from build123d import *

# Parameters (mm, degrees)
SKETCH2_W           = 236.22
SKETCH2_H           = 203.2
BOSS_EXTRUDE1_DEPTH = 3.175
SKETCH3_W           = 236.22
SKETCH3_H           = 3.175
BOSS_EXTRUDE2_DEPTH = 127
FILLET1_R           = 3.175
FILLET2_R           = 6.35


with BuildPart() as part:
    # Sketch2 → Boss-Extrude1 (new body)
    with BuildSketch(Plane.XY):
        Rectangle(SKETCH2_W, SKETCH2_H)
    extrude(amount=BOSS_EXTRUDE1_DEPTH)

    # Sketch3 → Boss-Extrude2 (add)
    with BuildSketch(Plane.XY.offset(3.175)):
        with Locations((0, -100.0125)):
            Rectangle(SKETCH3_W, SKETCH3_H)
    extrude(amount=BOSS_EXTRUDE2_DEPTH)

    # Fillet1
    fillet1_edges = [part.edges().sort_by_distance(p)[0] for p in [
        (0, -98.425, 3.175),
        (0, -101.6, 0),
    ]]
    fillet(fillet1_edges, radius=FILLET1_R)

    # Fillet2
    fillet2_edges = [part.edges().sort_by_distance(p)[0] for p in [
        (-118.11, -100.0125, 130.175),
        (118.11, -100.0125, 130.175),
        (-118.11, 101.6, 1.5875),
        (118.11, 101.6, 1.5875),
    ]]
    fillet(fillet2_edges, radius=FILLET2_R)


solid = part.part
Geometry: final body of the model. Coordinates: model frame, mm. A direction names the side the tool comes from. Give positions to 0.01 mm unless a question says otherwise; leave off trailing zeros. Write each loop counter-clockwise with the first axis right and the second up, starting at its lowest first coordinate (ties: lowest second). Pieces come first, ordered by that corner, then holes.
(1) Cut plane C-C, the plane y = 26.5. Return loops of the section in (x, z) (3 decimals).
(2) Cut plane B-B, the plane z = 23. Return loops of the section in (x, y) (3 decimals).
(3) Access query for faces 1 (the flat face through (-2, 5, 3.175)), 2 (the flat face through (118.11, -4, 2)). Directions: +Z, -Z, +X, -X, +Y, -Y. A direction counts if a zero-diameter tool reaches every point of the face in a straight line with its end or side. Return the directions, or none.
(4) First-contact query: P1, Ø2, axis at x = -10.5, z = 98, coming from the +Y side (3 decimals); P2, Ø2, axis at x = -25.5, y = 37.5, coming from the +Z side (3 decimals). Flat tips, straight axial feed; report the tip coordinate or a pass-through.
(5) Ray query, line 1 (Z direction, x = 91, y = -19) (3 decimals); line 2 (Y direction, x = 50.5, z = 90.5) (3 decimals). Return the intervals inside material, ascending.
(6) Cut plane A-A, the plane x = -34.5. Return loops of the section in (y, z) (3 decimals), then the cut area to 3 significant figures.
Values follow:
1. outline: (-118.11, 0) - (118.11, 0) - (118.11, 3.175) - (-118.11, 3.175) - close
2. outline: (-118.11, -101.6) - (118.11, -101.6) - (118.11, -98.425) - (-118.11, -98.425) - close
3. face 1: +Z, +X, -X, +Y
3. face 2: +Z, -Z, +X, +Y, -Y
4. P1: stops at y = -98.425
4. P2: stops at z = 3.175
5. line 1: z = 0 to 3.175
5. line 2: y = -101.6 to -98.425
6. outline: (-101.6, 3.175) arc R3.175 ccw to (-98.425, 0) - (101.6, 0) - (101.6, 3.175) - (-95.25, 3.175) arc R3.175 cw to (-98.425, 6.35) - (-98.425, 130.175) - (-101.6, 130.175) - close
6. area: 1,050 mm2
